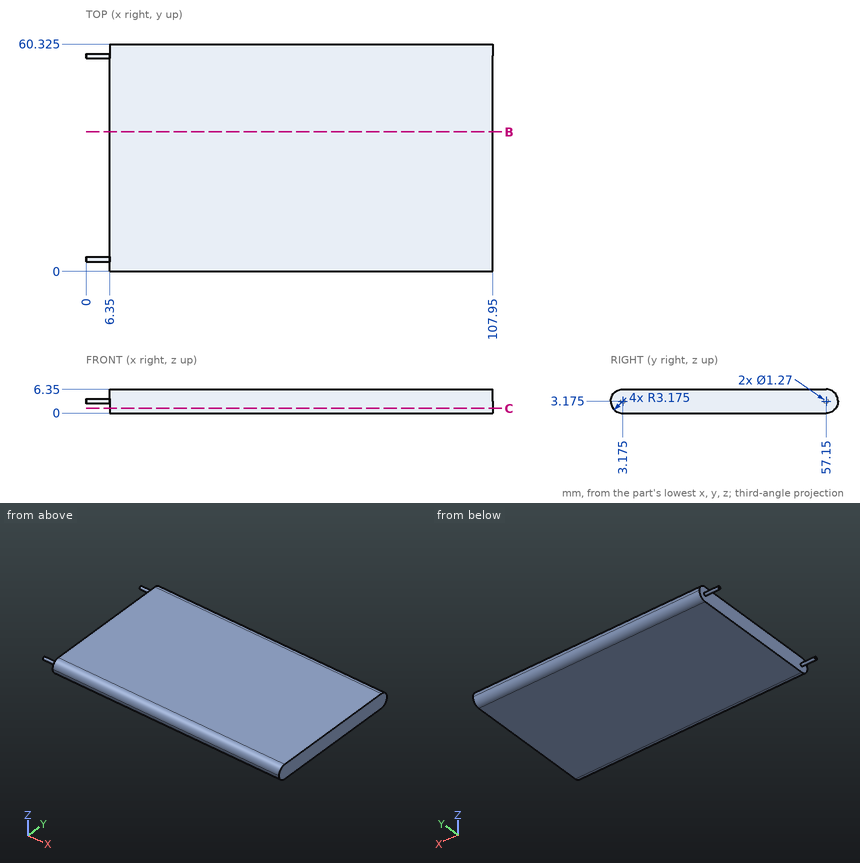
Study the drawing (mm; zero at the part's minimum x, y, z) and answer. Give positions to 0.01 mm unless a question says otherwise; leave off trailing zeros. Write each loop counter-clockwise with the first axis right and the second up, starting at its lowest first coordinate (ties: lowest second). Pieces come first, ordered by that corner, then holes. Notation, with made-up numbers: (-1, -28.75) -> (15, -28.75) arc R9 ccw to (15, -18.75) -> close; hole circle Ø3 at (77.25, 53). An arc over 180 degrees is marked (long way). Write item = value, one per line.
Q1. A flat-ended cylindrical pin translates along its axis: pin 1 Ø2 at (y, z) = (47, 4) entering from -X. Find the tip coordinate at first contact, or state that the pin passes through.
Computed values:
pin_1 = 6.35
Q2. Section B-B on y = 37 is taken. Determine the outline of the cut face in (x, z), and give its area (3 significant figures).
Computed values:
outline = (6.35, 0) -> (107.95, 0) -> (107.95, 6.35) -> (6.35, 6.35) -> close
area = 645 mm^2
Q3. Consider line 1 along X through (y, z) = (46.5, 0.5); line 2 along Y through (x, z) = (95.5, 3.75). Determine where each line is inside the solid, lowest interval first.
Computed values:
line_1 = 6.35 to 107.95
line_2 = 0.05 to 60.27
Q4. Section C-C on z = 1.25 is taken. Determine the outline of the cut face in (x, y) (3 decimals), and give its area (3 significant figures).
Computed values:
outline = (6.35, 0.65) -> (107.95, 0.65) -> (107.95, 59.675) -> (6.35, 59.675) -> close
area = 6,000 mm^2
